Check sheet for the modelled part. Datum: model origin and axes. Units: mm. A direction names the side the tool comes from. Round coordinates to 2 decimals unless told otherwise and drop trailing zeros. Loops run counter-clockwise (first coordinate to the right, second up) from the corner with the lowest first, then second, coordinate; pieces in that order, holes last. Notation, with made-up numbers: (-1, 61.5) - (53, 61.5) arc R16 ccw to (53, 67.5) - close; hole circle Ø10 at (18.25, -19). An arc over 180 degrees is marked (long way). Answer in a Markdown table with one row per item. Add a question column.
(1) Cross-section at D-D on y = 5.25. Enter the section's corners in (x, z).
(2) Cross-section at A-A on y = 0.5. Enter the section's corners in (x, z).
(3) Mould release check, pull along X, two halves, no side actions. Record for faces 1 (the cylindrical face through (-0.201, 6.147, 0.345)), 2 (the flat face through (0.1, 3.3, 0.7)), 3 (the cylindrical face through (3.62, 2.8, 0.35)): +X half, -X half, draft (parallel to the pull), parting line (faces both ways), or undercut.
(4) Cross-section at C-C on x = 0. Enter the section's corners in (y, z).
(5) Cross-section at B-B on x = -3.75. Enter the section's corners in (y, z).
(6) Thickness scan on line 1 along X through (y, z) = (3.5, 0.45); line 2 along Y through (x, z) = (3.5, 0.4); line 3 along X through (y, z) = (-1.5, 0.4). Record the ranges inside material, lowest first.
(7) Access from +Z, -Z, +X, -X, +Y, -Y to the whole of each face (thin tool, end or side, straight path). Record for faces 4 (the flat face through (0.1, 3.3, 0)), 5 (the flat face through (3.85, -3.71, 0.35)), 6 (the cylindrical face through (-3.64, 2.77, 0.35)).
Solid Edge part; units mm, degrees
sketch "Sketch1" plane through (0, 0, 0) normal (0, 0, 1) x (1, 0, 0)
  arc A0 (-4.1958, 1.8236) -> (-3, 0) centre (-3, 1.3039) ccw
  arc A1 (-2.65, -1.4062) -> (-3, 0) centre (0, 0) cw
  line L0 (-2.65, -1.4062) -> (-3.2938, -3.1751)
  line L1 (-3.2938, -3.1751) -> (-4.4278, -4.2682)
  arc A2 (-4.4278, -4.2682) -> (4.4278, -4.2682) centre (0, 0) cw
  line L2 (3.2938, -3.1751) -> (4.4278, -4.2682)
  line L3 (2.65, -1.4062) -> (3.2938, -3.1751)
  arc A3 (3, 0) -> (2.65, -1.4062) centre (0, 0) cw
  arc A4 (4.1958, 1.8236) -> (3, 0) centre (3, 1.3039) cw
  arc A5 (2.8475, 3.5809) -> (4.1958, 1.8236) centre (0, 0) cw
  arc A6 (2.8475, 3.5809) -> (0.7765, 2.8978) centre (2.0359, 2.5603) ccw
  arc A7 (-0.7765, 2.8978) -> (0.7765, 2.8978) centre (0, 0) cw
  arc A8 (-2.8475, 3.5809) -> (-0.7765, 2.8978) centre (-2.0359, 2.5603) cw
  arc A9 (-4.1958, 1.8236) -> (-2.8475, 3.5809) centre (0, 0) cw
extrude "Protrusion1" add sketch "Sketch1" along normal blind 0.7
properties material "Acier"
Answers:
| question | item | result |
|---|---|---|
| 1 | outline | (-3.2, 0) - (3.2, 0) - (3.2, 0.7) - (-3.2, 0.7) - close |
| 2 | outline | (-6.13, 0) - (-4.03, 0) - (-4.03, 0.7) - (-6.13, 0.7) - close; (4.03, 0) - (6.13, 0) - (6.13, 0.7) - (4.03, 0.7) - close |
| 3 | face 1 | parting line |
| 3 | face 2 | draft |
| 3 | face 3 | undercut |
| 4 | outline | (3, 0) - (6.15, 0) - (6.15, 0.7) - (3, 0.7) - close |
| 5 | outline | (-3.61, 0) - (0.24, 0) - (0.24, 0.7) - (-3.61, 0.7) - close; (2.62, 0) - (4.87, 0) - (4.87, 0.7) - (2.62, 0.7) - close |
| 6 | line 1 | x = -5.06 to -2.95, -1.13 to 1.13, 2.95 to 5.06 |
| 6 | line 2 | y = -3.37 to 0.1, 2.95 to 5.06 |
| 6 | line 3 | x = -5.96 to -2.68, 2.68 to 5.96 |
| 7 | face 4 | -Z, +X, -X, +Y, -Y |
| 7 | face 5 | +Z, -Z, -Y |
| 7 | face 6 | +Z, -Z |
